Design review of the part built by this model. Coordinates are the model's own, in mm. A direction names the side the tool comes from. Round coordinates to 2 decimals unless told otherwise and drop trailing zeros. Write each loop counter-clockwise with the first axis right and the second up, starting at its lowest first coordinate (ties: lowest second). Pieces come first, ordered by that corner, then holes. Notation, with made-up numbers: M 21.5,42.25 L 25.5,42.25 A23 cw 25.5,60.25 Z; hole C 2.5,48 d4. An arc over 180 degrees is marked long. Use CSV: the item, a comma, the result in double quotes.
from build123d import *

# Parameters (mm, degrees)
BOSS_EXTRUDE1_DEPTH = 10
SKETCH3_W           = 5
SKETCH3_H           = 1.75
BOSS_EXTRUDE2_DEPTH = 90
SKETCH4_R           = 1.5
CUT_EXTRUDE1_DEPTH  = 111


with BuildPart() as part:
    # Sketch1 → Boss-Extrude1 (new body)
    with BuildSketch(Plane.XY):
        Polygon((0, 10.81190481), (0, -9.18809519), (15, -9.18809519), (15, -4.18809519), (5, -4.18809519), (5, 5.81190481), (15, 5.81190481), (15, 10.81190481), align=None)
    extrude(amount=BOSS_EXTRUDE1_DEPTH)

    # Sketch3 → Boss-Extrude2 (add)
    with BuildSketch(Plane(origin=(0, -9.18809519, 0), x_dir=(-1, 0, 0), z_dir=(0, -1, 0))):
        with Locations((-12.5, -0.875)):
            Rectangle(SKETCH3_W, SKETCH3_H)
    extrude(amount=BOSS_EXTRUDE2_DEPTH)

    # Sketch4 → Cut-Extrude1 (cut, through all)
    with BuildSketch(Plane(origin=(0, 10.81190481, 0), x_dir=(1, 0, 0), z_dir=(0, 1, 0))):
        with Locations((7.5, -5)):
            Circle(SKETCH4_R)
    extrude(amount=-CUT_EXTRUDE1_DEPTH, mode=Mode.SUBTRACT)


solid = part.part
1) Add section B-B on z = 5. Write out the cut boundary in (x, y), then the cut area to 3 significant figures.
Answers:
outline,"M 0,-9.19 L 6,-9.19 L 6,-4.19 L 5,-4.19 L 5,5.81 L 6,5.81 L 6,10.81 L 0,10.81 Z; M 9,-9.19 L 15,-9.19 L 15,-4.19 L 9,-4.19 Z; M 9,5.81 L 15,5.81 L 15,10.81 L 9,10.81 Z"
area,"170 mm²"
2) Machinability: for faces 1 (the face through (4, 1, 10)), 2 (the face through (5, 1, 5)), 3 (the face through (10, -54, 1)), 4 (the face through (13, -54, 1.75)), which of the approach directions +Z, -Z, +X, -X, +Y, -Y give a long, thin tool a straight path to every point of the face, cutting with its end or side? Answer none if there is none.
Answers:
face 1,"+Z, +X, -X, +Y, -Y"
face 2,"+Z, -Z, +X"
face 3,"+Z, -Z, -X, -Y"
face 4,"+Z, +X, -X, -Y"
3) For pin 1 Ø3 at (x, y) = (12.5, -30) entering from -Z; pin 2 Ø3 at (y, z) = (-1.5, 4.5) entering from +X; pin 3 Ø5 at (x, z) = (11.5, 7) entering from -Y; pin 4 Ø0.9 at (y, z) = (-37.5, 1.5) entering from -X, all flat-tipped, find the tip position at first contact; note any pin that passes through.
Answers:
pin 1,"z = 0"
pin 2,"x = 5"
pin 3,"y = -9.19"
pin 4,"x = 10"
4) Add section C-C on x = 7.25. Write out the cut boundary in (y, z).
Answers:
outline,"M -9.19,0 L -4.19,0 L -4.19,3.52 L -9.19,3.52 Z; M -9.19,6.48 L -4.19,6.48 L -4.19,10 L -9.19,10 Z; M 5.81,0 L 10.81,0 L 10.81,3.52 L 5.81,3.52 Z; M 5.81,6.48 L 10.81,6.48 L 10.81,10 L 5.81,10 Z"
5) Wall thickness on line 1 along Z through (x, y) = (7.5, -6.65); line 2 along X through (y, z) = (7, 5); line 3 along Y through (x, z) = (7.5, 8.5): over which ranges is each line inside the solid? List them lowest first. Write a range as [from, to].
Answers:
line 1,"[0, 3.5], [6.5, 10]"
line 2,"[0, 6], [9, 15]"
line 3,"[-9.19, -4.19], [5.81, 10.81]"
6) The part is to be moulded in two halves that separate along X. For faces 5 (the face through (11, -31, 0)), 6 (the face through (6.39, 8.35, 3.99)), 7 (the face through (15, 8, 5)), 8 (the face through (6.39, -6.65, 3.99)), say which applies: released by +X, released by -X, zero draft, split by the parting line, or undercut.
Answers:
face 5,"zero draft"
face 6,"undercut"
face 7,"released by +X"
face 8,"undercut"
7) Add section A-A on x = 11.25. Write out the cut boundary in (y, z), then the cut area to 4 significant figures.
Answers:
outline,"M -99.19,0 L -4.19,0 L -4.19,10 L -9.19,10 L -9.19,1.75 L -99.19,1.75 Z; M 5.81,0 L 10.81,0 L 10.81,10 L 5.81,10 Z"
area,"257.5 mm²"
8) Add section D-D on y = -68. Write out the cut boundary in (x, z).
Answers:
outline,"M 10,0 L 15,0 L 15,1.75 L 10,1.75 Z"
